Work out the finished part from the listing and answer in its coordinate system (mm). Face numbers are marked on the shaded views. A direction names the side the tool comes from. Round coordinates to 2 decimals unless told otherwise and drop trailing zeros. Write each loop counter-clockwise with the first axis right and the second up, starting at its lowest first coordinate (ties: lowest second). Pieces come first, ordered by that corner, then holes. Notation, with made-up numbers: (-12.75, 76) - (21.25, 76) arc R10 ccw to (21.25, 89) - close; hole circle Ø5 at (-29.5, 83). An arc over 180 degrees is marked (long way). Answer as a JSON object with one key per item and string values.
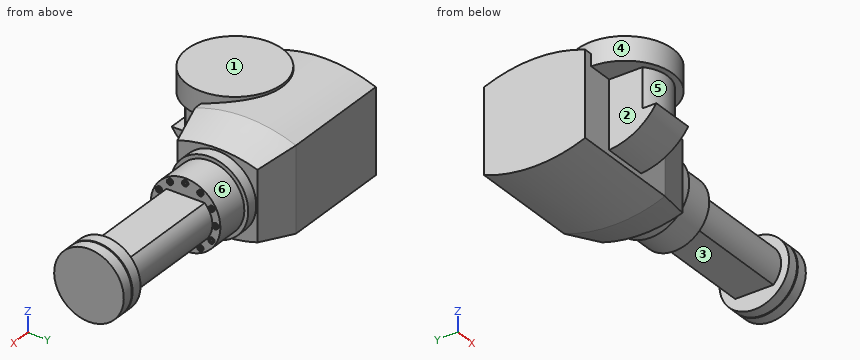
Autodesk Fusion 360 part; units mm, degrees
sketch "Sketch1" plane through (0, 0, 0) normal (1, 0, 0) x (0, 0, -1)
  line L0 (0, 0) -> (0, 45)
  line L1 (0, 0) -> (0, -45)
  line L2 (0, 45) -> (37.5, 45)
  line L3 (0, 45) -> (-37.5, 45)
  line L4 (0, -45) -> (37.5, -45)
  line L5 (0, -45) -> (-37.5, -45)
  arc A0 (-37.5, 45) -> (-37.5, -45) centre (79.119, 0) ccw
  arc A1 (37.5, -45) -> (37.5, 45) centre (-79.119, 0) ccw
  dimension "d1" = 45
  dimension "d2" = 45
  dimension "d3" = 37.5
  dimension "d4" = 37.5
  dimension "d5" = 37.5
  dimension "d6" = 37.5
  dimension "d8" = 125
extrude "Extrude1" add sketch "Sketch1" along normal blind 100
extrude "Extrude2" add 1 faces at (100, -15.2642, -14.2806) along direction (1, 0, 0) blind 35 draft -15
sketch "Sketch2" plane through (135, 0, 0) normal (1, 0, 0) x (0, 0, -1)
  line L0 (-30.8786, -35.6218) -> (30.8786, -35.6218)
  arc A0 (30.8786, -35.6218) -> (30.8786, 35.6218) centre (-79.119, 0) ccw
  line L1 (30.8786, 35.6218) -> (-30.8786, 35.6218)
  arc A1 (-30.8786, 35.6218) -> (-30.8786, -35.6218) centre (79.119, 0) ccw
  circle A2 centre (0, 0) radius 34.5
  dimension "d13" = 69
extrude "Extrude3" add sketch "Sketch2" along normal blind 10 contours A2
sketch "Sketch3" plane through (145, 0, 0) normal (1, 0, 0) x (0, 0, -1)
  circle A0 centre (0, 0) radius 34.5
  circle A1 centre (0, 0) radius 31
  dimension "d16" = 62
extrude "Extrude4" add sketch "Sketch3" along normal blind 30 contours A1
sketch "Sketch4" plane through (175, 0, 0) normal (1, 0, 0) x (0, 0, -1)
  circle A0 centre (0, 0) radius 31
  line L0 (0, 0) -> (27, 0)
  circle A1 centre (27, 0) radius 2.5
  circle A2 centre (27, 0) radius 1.5
  dimension "d19" = 27
  dimension "d20" = 5
  dimension "d21" = -1
extrude "Extrude5" add sketch "Sketch4" along normal blind 1 contours A1
pattern_circular "C-Pattern1" count 12 over 360 about axis through (175, 0, 0) along (1, 0, 0) of "Extrude5"
sketch "Sketch5" plane through (175, 0, 0) normal (1, 0, 0) x (0, 0, -1)
  circle A0 centre (27, 0) radius 2.5
  circle A1 centre (0, 0) radius 31
  circle A2 centre (23.3827, 13.5) radius 2.5
  circle A3 centre (13.5, 23.3827) radius 2.5
  circle A4 centre (0, 27) radius 2.5
  circle A5 centre (-13.5, 23.3827) radius 2.5
  circle A6 centre (-23.3827, 13.5) radius 2.5
  circle A7 centre (-27, 0) radius 2.5
  circle A8 centre (-23.3827, -13.5) radius 2.5
  circle A9 centre (-13.5, -23.3827) radius 2.5
  circle A10 centre (0, -27) radius 2.5
  circle A11 centre (13.5, -23.3827) radius 2.5
  circle A12 centre (23.3827, -13.5) radius 2.5
  line L0 (0, 0) -> (16, 0)
  line L1 (16, 0) -> (16, 17)
  line L2 (16, 0) -> (16, -17)
  line L3 (0, 0) -> (0, -8.0593)
  line L4 (-16, 0) -> (-16, 17)
  line L5 (-16, 0) -> (-16, -17)
  arc A13 (16, 17) -> (-16, 17) centre (0, 1.9003) ccw
  arc A14 (-16, -17) -> (16, -17) centre (0, -1.9003) ccw
  dimension "d26" = 16
  dimension "d27" = 17
  dimension "d28" = 17
  dimension "d29" = 22
extrude "Extrude6" add sketch "Sketch5" along normal blind 100 contours L1 L2 L4 L5 A13 A14
sketch "Sketch6" plane through (275, 0, 0) normal (1, 0, 0) x (0, 0, -1)
  line L0 (-16, 17) -> (-16, -17)
  arc A0 (-16, -17) -> (16, -17) centre (0, -1.9003) ccw
  line L1 (16, -17) -> (16, 17)
  arc A1 (16, 17) -> (-16, 17) centre (0, 1.9003) ccw
  circle A2 centre (0, 0) radius 31
  circle A3 centre (0, 0) radius 30
  dimension "d32" = 62
  dimension "d35" = -1
extrude "Extrude7" add sketch "Sketch6" along normal blind 10 contours L0 A0 L1 A1 | A2 | A3
sketch "Sketch7" plane through (285, 0, 0) normal (1, 0, 0) x (0, 0, -1)
  circle A0 centre (0, 0) radius 31
  circle A1 centre (0, 0) radius 30
  dimension "d36" = -1
extrude "Extrude8" add sketch "Sketch7" along normal blind 1 contours A1
sketch "Sketch8" plane through (286, 0, 0) normal (1, 0, 0) x (0, 0, -1)
  circle A0 centre (0, 0) radius 30
  circle A1 centre (0, 0) radius 31
  dimension "d39" = 62
extrude "Extrude9" add sketch "Sketch8" along normal blind 10 contours A0 | A1
ref_plane "WorkPlane1" through (0, 45, 37.5) normal (0, 0, 1) x (1, 0, 0)
sketch "Sketch9" plane through (0, 0, 37.5) normal (0, 0, 1) x (1, 0, 0)
  circle A0 centre (50, -45) radius 42.5
  dimension "d43" = 85
extrude "Extrude10" add sketch "Sketch9" along normal mid plane 21
sketch "Sketch10" plane through (0, 0, 27) normal (0, 0, -1) x (-1, 0, 0)
  line L0 (-7.5, -45) -> (-92.5, -45)
  arc A0 (-92.5, -45) -> (-7.5, -45) centre (-50, -45) ccw
  line L1 (-50, -45) -> (-50, -75)
  line L2 (-70, -45) -> (-70, -74.9351)
  line L3 (-30, -45) -> (-30, -74.738)
  arc A1 (-70, -74.9351) -> (-30, -74.738) centre (-50.1102, -52.4763) ccw
  dimension "d46" = 30
  dimension "d47" = 20
  dimension "d48" = -20
  dimension "d49" = 30
extrude "Extrude11" add sketch "Sketch10" along normal blind 35 contours L0 L2 L3 A1
sketch "Sketch11" plane through (70, 0, 0) normal (1, 0, 0) x (0, 0, -1)
  line L0 (-27, -45) -> (-27, -74.9351)
  line L1 (-27, -74.9351) -> (8, -74.9351)
  line L2 (8, -74.9351) -> (8, -45)
  line L3 (8, -45) -> (-27, -45)
  line L4 (8, -45) -> (33, -45)
  arc A0 (8, -87) -> (33, -45) centre (-21.8393, -40.7981) ccw
  line L5 (8, -45) -> (8, -87)
  dimension "d52" = 25
  dimension "d54" = 55
extrude "Extrude12" add sketch "Sketch11" against normal blind 40 contours L2 L4 A0 L5
equation "d44 = ( 21 / 2 ) * 1 mm"
Item 1: A cutting plane is placed at C-C (x = 156). Write down the section's boundary in (y, z).
Results found:
{"outline": "circle Ø62 at (0, 0)"}
Item 2: A cutting plane is placed at B-B (x = 249.5). Write down the section's boundary in (y, z), and give its area (3 significant figures).
Results found:
{"outline": "(-17, -16) - (17, -16) arc R22 ccw to (17, 16) - (-17, 16) arc R22 ccw to start", "area": "1,390 mm²"}
Item 3: A cutting plane is placed at A-A (x = 82). Write down the section's boundary in (y, z), and give its area (3 significant figures).
Results found:
{"outline": "(-72.97, 27) - (-45, 27) - (-45, -37.5) arc R125 ccw to (45, -37.5) - (45, 37.5) arc R125 ccw to (-17.03, 44.72) - (-17.03, 48) - (-72.97, 48) - close", "area": "8,530 mm²"}
Item 4: A cutting plane is placed at D-D (x = 50). Write down the section's boundary in (y, z), and give its area (3 significant figures).
Results found:
{"outline": "(-87.5, 27) - (-82.48, 27) - (-82.48, -8) - (-87, -8) arc R55 ccw to (-45, -33) - (-45, -37.5) arc R125 ccw to (45, -37.5) - (45, 37.5) arc R125 ccw to (-2.5, 45.86) - (-2.5, 48) - (-87.5, 48) - close", "area": "10,900 mm²"}
Item 5: Consider line 1 along Z through (x, y) = (175.35, -13.5); line 2 along Z through (x, y) = (175.75, 0); line 3 along X through (y, z) = (23, -14). Determine where each line is inside the solid, lowest interval first.
Results found:
{"line 1": "-25.88 to -24.88, -21.88 to -20.88, -16 to 16, 20.88 to 21.88, 24.88 to 25.88", "line 2": "-29.5 to -28.5, -25.5 to -24.5, -16 to 16, 24.5 to 25.5, 28.5 to 29.5", "line 3": "0 to 175, 275 to 296"}
Item 6: Determine the mould class of the marked faces 1, 2 and 3 for opening direction X: pulls with the +X half, pulls with the -X half, needs draft (parallel to the pull), parting line crosses it, or undercut.
Results found:
{"face 1": "needs draft", "face 2": "pulls with the -X half", "face 3": "undercut"}
Item 7: Each of these flat-tipped pins is pushed along its axis until it touches: P1, Ø2, axis at x = 212.5, y = -19.5, coming from the +Z side; P2, Ø12, axis at x = 245.5, y = -31.5, coming from the -Z side; P3, Ø5, axis at x = 145, y = 19.5, coming from the -Z side; P4, Ø2, axis at x = 92, z = 3, coming from the -Y side. Where does it stop, or does it pass through?
Results found:
{"P1": "z = 14.44", "P2": "through", "P3": "z = -30.02", "P4": "y = -45"}
Item 8: For the marked faces 4, 5 and 6, determine the directions among +Z, -Z, +X, -X, +Y, -Y from which every point of the face is accessible in a straight line to the end or side of a thin tool.
Results found:
{"face 4": "+Z", "face 5": "-Y", "face 6": "+X"}
